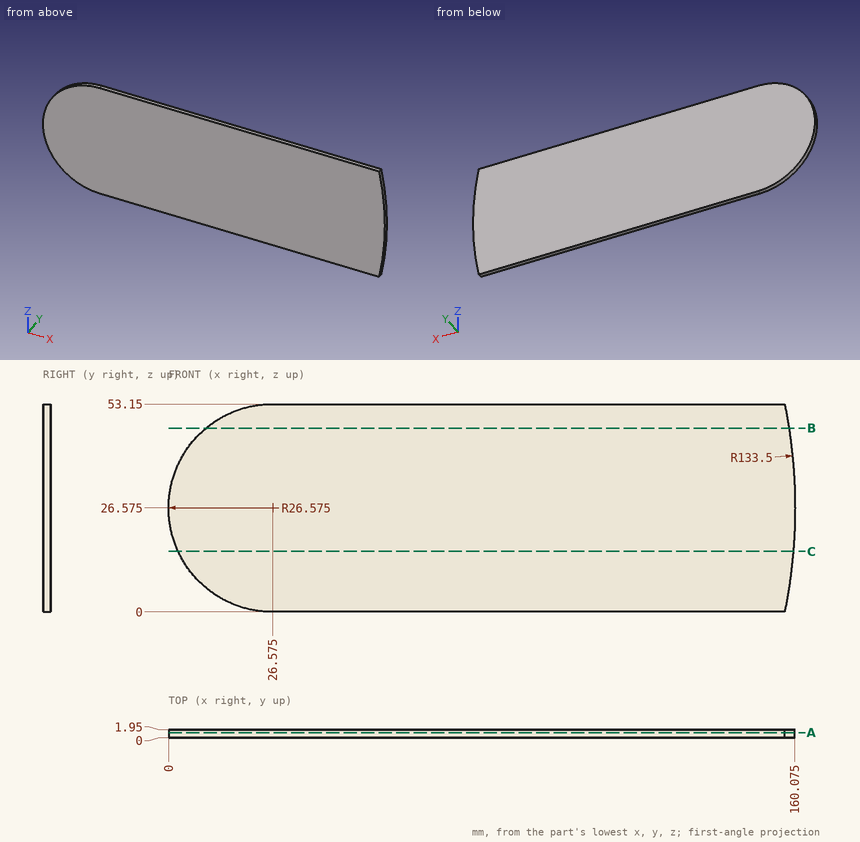
Here's the drawing with two shaded views (mm, measured from the low corner). I have some questions. Give positions to 0.01 mm unless a question says otherwise; leave off trailing zeros. Loops run counter-clockwise (first coordinate to the right, second up) from the corner with the lowest first, then second, coordinate; pieces in that order, holes last. Notation, with made-up numbers: (32, 36.25) -> (75, 36.25) arc R24 ccw to (75, 55.25) -> close; hole circle Ø4 at (57.25, 15). An arc over 180 degrees is marked (long way). Answer as a JSON object with one key per item and string values. Group by question number.
Item 1: I need wall thicknesses on L1, parallel to Z at x = 7, y = 1.85; L2, parallel to X at y = 0.1, z = 37.5; L3, parallel to X at y = 0.4, z = 14.5. Which ranges of each line are inside material? Lowest first, please.
Item 2: Imagine slicing it at B-B on z = 47. Write out the boundary of the cut face in (x, y).
Item 3: Will these pins go through, and if not, where does the flat tip stop? pin 1 (1 mm diameter, centred on y = 1, z = 7, fed in from -X); pin 2 (1 mm diameter, centred on x = 119, z = 9.5, fed in from -Y).
Item 4: Imagine slicing it at C-C on z = 15.5. Write out the boundary of the cut face in (x, y).
Item 5: Imagine slicing it at A-A on y = 1.25. Write out the boundary of the cut face in (x, z) (3 decimals).
Answer list:
{
 "1": {"L1": "z = 8.6 to 44.55", "L2": "x = 2.35 to 159.63", "L3": "x = 2.9 to 159.53"},
 "2": {"outline": "(9.57, 0) -> (158.5, 0) -> (158.5, 1.95) -> (9.57, 1.95) -> close"},
 "3": {"pin 1": "stops at x = 8.07", "pin 2": "stops at y = 0"},
 "4": {"outline": "(2.42, 0) -> (159.61, 0) -> (159.61, 1.95) -> (2.42, 1.95) -> close"},
 "5": {"outline": "(26.575, 0) -> (157.403, 0) arc R133.5 ccw to (157.403, 53.15) -> (26.575, 53.15) arc R26.575 ccw to start"}
}
